Here's how the part is built. I have some questions about the finished solid (model axes, mm). A direction names the side the tool comes from. Round coordinates to 2 decimals unless told otherwise and drop trailing zeros. Order: outer loops, then holes, each group sorted by start corner. A loop starts at its lowest first (then second) coordinate and runs counter-clockwise, first axis right, second up. Notation, with made-up numbers: M -32.5,31 L -13.5,31 A16 cw -13.5,46 Z; hole C -39.5,-25.75 d2. An arc over 180 degrees is marked long. Answer as CSV lines item,"result". Start each with the question number.
```python
from build123d import *

# Parameters (mm, degrees)
SKETCH1_R           = 34.5
SKETCH1_R_2         = 4
BOSS_EXTRUDE1_DEPTH = 5
CUT_EXTRUDE2_DEPTH  = 50.045896872
CIRPATTERN1_COUNT   = 4


with BuildPart() as part:
    # Sketch1 → Boss-Extrude1 (new body)
    with BuildSketch(Plane(origin=(0, 0, 0), x_dir=(1, 0, 0), z_dir=(0, 1, 0))):
        with Locations(Location((0, 0, 0), (0, 0, 270))):
            Circle(SKETCH1_R)
        with Locations(Location((0, 0, 0), (0, 0, 270))):
            Circle(SKETCH1_R_2, mode=Mode.SUBTRACT)
    extrude(amount=BOSS_EXTRUDE1_DEPTH)

    # Sketch8 → Cut-Extrude2 (cut, through all)
    with BuildSketch(Plane(origin=(0, 5, 0), x_dir=(1, 0, 0), z_dir=(0, 1, 0))):
        with BuildLine():
            Line((-8.698076686, -2), (-28.201327726, -2))
            ThreePointArc((-28.201327726, -2), (-29.040208751, -2.374920589), (-29.320428032, -3.25))
            ThreePointArc((-29.320428032, -3.25), (-20.856955891, -20.862343851), (-3.242426547, -29.321266516))
            ThreePointArc((-3.242426547, -29.321266516), (-2.372627527, -29.04255234), (-2, -28.208657471))
            Line((-2, -28.208657471), (-2, -8.645966692))
            ThreePointArc((-2, -8.645966692), (-2.222589282, -7.955091785), (-2.787089084, -7.498808868))
            Line((-2.787089084, -7.498808868), (-2.857385295, -7.472305486))
            ThreePointArc((-2.857385295, -7.472305486), (-5.662928364, -5.650773606), (-7.478427834, -2.841323131))
            ThreePointArc((-7.478427834, -2.841323131), (-7.957237983, -2.230732861), (-8.698076686, -2))
        make_face()
    cut_extrude2 = extrude(amount=-CUT_EXTRUDE2_DEPTH, mode=Mode.SUBTRACT)

    # CirPattern1: Cut-Extrude2 ×4 about axis
    cirpattern1_axis = Axis((0, 0, 0), (0, 1, 0))
    for i in range(1, CIRPATTERN1_COUNT):
        add(cut_extrude2.rotate(cirpattern1_axis, i * 360 / CIRPATTERN1_COUNT), mode=Mode.SUBTRACT)


solid = part.part
```
Item 1: If I drill on line 1 along X through (y, z) = (3.9, 0); line 2 along X through (y, z) = (2.95, -16); line 3 along Z through (x, y) = (-15.5, 4.25), over which ranges is the centre line in solid material (lowest first)?
Item 2: If we section it at C-C on z = 0: Please give me the cut outline in (x, y), and give its area (3 significant figures).
Item 3: If we section it at D-D on x = -10: Please give me the cut outline in (y, z), and give its area (3 significant figures).
Item 4: If we section it at B-B on z = -20: Please give me the cut outline in (x, y), and give its area (3 significant figures).
Item 5: If we section it at A-A on x = 0: Please give me the cut outline in (y, z), and give its area (3 significant figures).
Item 6: We'd pull the mould along X, two halves only. Please class faces 3 (the cylindrical face through (1.517, 2.465, -34.467)), 4 (the cylindrical face through (5.684, 2.535, 5.63)), 5 (the flat face through (-7, 5, 0)): pulls with the +X half, pulls with the -X half, needs draft (parallel to the pull), parting line crosses it, or undercut.
Item 7: For P1, Ø1, axis at x = -20.5, y = 0.5, coming from the -Z side; P2, Ø1, axis at y = 2.5, z = 2.5, coming from the -X side; P3, Ø3, axis at x = 9.5, y = 0.5, coming from the +Z side; P4, Ø7, axis at x = 0, z = 0, coming from the -Y side, each with a flat end and sliding along its axis, tell me the tip position at first contact or that it passes through.
Item 8: Which directions (+Z, -Z, +X, -X, +Y, -Y) give clear straight access to the entire face, cutting with the end or side of a thin tool? Please do faces 1 (the flat face through (-2, 3, 19)), 2 (the flat face through (-7, 0, 0)).
Geometry says:
1,line 1,"-34.5 to -4, 4 to 34.5"
1,line 2,"-30.57 to -24.78, -2 to 2, 24.78 to 30.57"
1,line 3,"-30.82 to -25.1, -2 to 2, 25.1 to 30.82"
2,outline,"M -34.5,0 L -4,0 L -4,5 L -34.5,5 Z; M 4,0 L 34.5,0 L 34.5,5 L 4,5 Z"
2,area,"305 mm²"
3,outline,"M 0,-33.02 L 5,-33.02 L 5,-27.75 L 0,-27.75 Z; M 0,-2 L 5,-2 L 5,2 L 0,2 Z; M 0,27.75 L 5,27.75 L 5,33.02 L 0,33.02 Z"
3,area,"72.7 mm²"
4,outline,"M -28.11,0 L -21.69,0 L -21.69,5 L -28.11,5 Z; M -2,0 L 2,0 L 2,5 L -2,5 Z; M 21.69,0 L 28.11,0 L 28.11,5 L 21.69,5 Z"
4,area,"84.3 mm²"
5,outline,"M 0,-34.5 L 5,-34.5 L 5,-4 L 0,-4 Z; M 0,4 L 5,4 L 5,34.5 L 0,34.5 Z"
5,area,"305 mm²"
6,face 3,"parting line crosses it"
6,face 4,"undercut"
6,face 5,"needs draft"
7,P1,"z = -28.11"
7,P2,"x = -34.44"
7,P3,"z = 33.56"
7,P4,"through"
8,face 1,"+Y, -Y"
8,face 2,"+Z, -Z, +X, -X, -Y"
